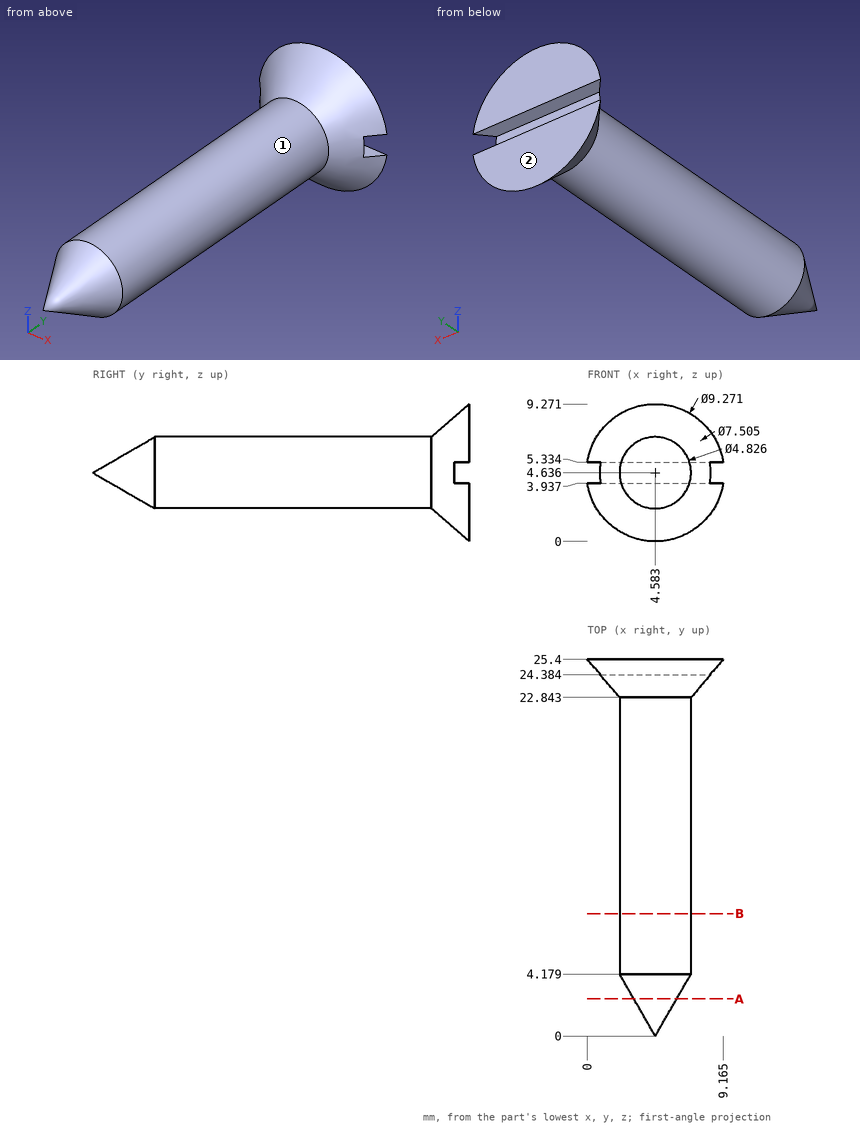
Print and shaded views of the part. All mm, measured from the part's lowest x, y and z. A direction names the side the tool comes from. Give positions to 0.01 mm unless a question says otherwise; leave off trailing zeros. Order: outer loops, then holes, each group sorted by start corner. A loop starts at its lowest first (then second) coordinate and runs counter-clockwise, first axis right, second up. Notation, with made-up numbers: (-20, 27.5) - (-8, 27.5) arc R15 ccw to (-8, 40.5) - close; hole circle Ø6 at (22, 44.5). An arc over 180 degrees is marked (long way). Use a Markdown table: item, result.
1) Flat gauge pins, fed straight in: P1, Ø4, axis at x = 5.5, y = 13, coming from the -Z side; P2, Ø1.1, axis at x = 5.5, y = 25, coming from the +Z side; P3, Ø1, axis at x = 6, y = 5, coming from the +Z side. Where does each tip first touch, or does it go through?
Checked values:
| item | result |
|---|---|
| P1 | z = 2.22 |
| P2 | z = 9.24 |
| P3 | z = 6.87 |
2) Probe L1, parallel to X at y = 11.5, z = 4.75; L2, parallel to Y at x = 5.25, z = 4.5 (1 decimal); L3, parallel to Y at x = 6, z = 6.25. List the from-to ranges inside material, lowest first. Write a range as from..to.
Checked values:
| item | result |
|---|---|
| L1 | 2.17..6.99 |
| L2 | 1.2..24.4 |
| L3 | 3.72..25.4 |
3) 3-axis set-ups, long thin cutter, end or side, ignore diameter. For the marked faces 1 and 2: which of +Z, -Z, +X, -X, +Y, -Y reach the whole face in a straight line?
Checked values:
| item | result |
|---|---|
| face 1 | -Y |
| face 2 | +Z, -Z, +X, -X, +Y |
4) Saw through at A-A on y = 2.5. List the corners of the cut face in (x, z) (1 decimal).
Checked values:
| item | result |
|---|---|
| outline | circle Ø2.9 at (4.6, 4.6) |
5) Saw through at B-B on y = 8.25. List the corners of the cut face in (x, z) (1 decimal).
Checked values:
| item | result |
|---|---|
| outline | circle Ø4.8 at (4.6, 4.6) |
